from build123d import *

# Parameters (mm, degrees)
SKETCH1_R           = 1.47
BOSS_EXTRUDE1_DEPTH = 1.5875
SKETCH3_R           = 1.0287
CUT_EXTRUDE1_DEPTH  = 4.175


with BuildPart() as part:
    # Sketch1 → Boss-Extrude1 (new body, symmetric)
    with BuildSketch(Plane.XY):
        Polygon((-12.5, 60), (-70, 60), (-70, 12.5), (-73.175, 12.5), (-73.175, -12.5), (-70, -12.5), (-70, -60), (-12.5, -60), (-12.5, -56.825), (-1.47, -56.825), (-1.47, -53.125), (-3.25, -53.125), (-3.25, -50.525), (-1.47, -50.525), (-1.47, -46.825), (1.47, -46.825), (1.47, -50.525), (3.25, -50.525), (3.25, -53.125), (1.47, -53.125), (1.47, -56.825), (12.5, -56.825), (12.5, -60), (70, -60), (70, -12.5), (73.175, -12.5), (73.175, 12.5), (70, 12.5), (70, 60), (12.5, 60), (12.5, 56.825), (1.47, 56.825), (1.47, 53.125), (3.25, 53.125), (3.25, 50.525), (1.47, 50.525), (1.47, 46.825), (-1.47, 46.825), (-1.47, 50.525), (-3.25, 50.525), (-3.25, 53.125), (-1.47, 53.125), (-1.47, 56.825), (-12.5, 56.825), align=None)
        with Locations((-71.5875, 0)):
            Circle(SKETCH1_R, mode=Mode.SUBTRACT)
        with Locations((71.5875, 0)):
            Circle(SKETCH1_R, mode=Mode.SUBTRACT)
    extrude(amount=BOSS_EXTRUDE1_DEPTH, both=True)

    # Sketch3 → Cut-Extrude1 (cut, through all)
    with BuildSketch(Plane(origin=(0, 0, -1.5875), x_dir=(-1, 0, 0), z_dir=(0, 0, -1))):
        with Locations((-51.375, -23.975)):
            Circle(SKETCH3_R)
        with Locations((-52.975, 24.325)):
            Circle(SKETCH3_R)
        with Locations((-0.575, -8.675)):
            Circle(SKETCH3_R)
        with Locations((-0.575, 19.225)):
            Circle(SKETCH3_R)
    extrude(amount=-CUT_EXTRUDE1_DEPTH, mode=Mode.SUBTRACT)


solid = part.part
Work out the finished part from the listing and answer in its coordinate system (mm). A direction names the side the tool comes from. Coordinates: 2 decimals unless noted, no trailing zeros. Write each loop counter-clockwise with the first axis right and the second up, starting at its lowest first coordinate (ties: lowest second). Pieces come first, ordered by that corner, then holes. Notation, with made-up numbers: M 45.5,68.25 L 101.5,68.25 A19 cw 101.5,102.25 Z; hole C -4,-23 d2. An arc over 180 degrees is marked long. Answer as CSV lines item,"result". Start each with the question number.
Item 1: Consider L1, parallel to X at y = 53.5, z = 0.2; L2, parallel to X at y = -51, z = -0.5; L3, parallel to X at y = 17, z = 0.3. Determine where each line is inside the solid, lowest interval first.
Item 2: A tool of negligible diameter and unlimited length cuts with its end or side. For faces 4 (the face through (72, 12.5, 0)), 5 (the face through (-1.47, 49, 0)), 6 (the face through (-1, 1, -1.588)), 7 (the face through (7, -56.825, 0)), 8 (the face through (-72, -12.5, 0)), from which of +Z, -Z, +X, -X, +Y, -Y can it reach the whole face along a straight path? Write none if from no direction.
Item 3: Determine the mould class of faces 1 (the face through (-70, -36, 0)), 2 (the face through (70.12, 0.06, -0.02)), 3 (the face through (-72, 12.5, 0)) for opening direction X: released by +X, released by -X, zero draft, split by the parting line, or undercut.
Item 4: Section C-C on x = -6.5 is taken. Write down the section's boundary in (y, z) (1 decimal), and give its area (3 significant figures).
Item 5: Section B-B on z = -0.3 is taken. Give the number of separate pieces and of enclosed holes in the cut face, and give its area (3 significant figures).
Item 6: Flat-ended cylindrical pins translate along their axes: P1, Ø1, axis at y = 59, z = -0.5, coming from the +X side; P2, Ø1.6, axis at x = 72, z = 0.5, coming from the +Y side; P3, Ø1, axis at y = -15, z = 1, coming from the -X side. Find the tip coordinate at first contact, or state that the pin passes through.
Item 7: Section A-A on y = 29.5 is taken. Write down the section's boundary in (x, z), and give its area (4 significant figures).
Checks:
1,L1,"x = -70 to -1.47, 1.47 to 70"
1,L2,"x = -70 to -3.25, 3.25 to 70"
1,L3,"x = -70 to 70"
2,face 4,"+Z, -Z, +X, +Y"
2,face 5,"+Z, -Z, +Y"
2,face 6,"-Z, +X, -X, +Y, -Y"
2,face 7,"+Z, -Z, -Y"
2,face 8,"+Z, -Z, -X, -Y"
3,face 1,"released by -X"
3,face 2,"undercut"
3,face 3,"zero draft"
4,outline,"M -56.8,-1.6 L 56.8,-1.6 L 56.8,1.6 L -56.8,1.6 Z"
4,area,"361 mm²"
5,separate pieces,"1"
5,enclosed holes,"6"
5,area,"16,700 mm²"
6,P1,"stops at x = 70"
6,P2,"stops at y = 12.5"
6,P3,"stops at x = -70"
7,outline,"M -70,-1.59 L 70,-1.59 L 70,1.59 L -70,1.59 Z"
7,area,"444.5 mm²"
